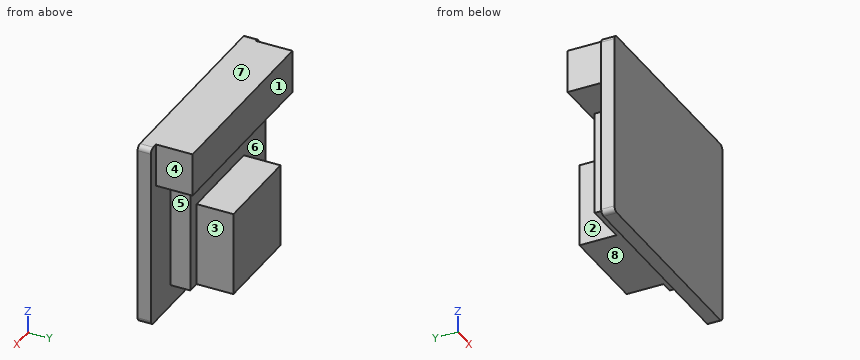
```python
from build123d import *

# Parameters (mm, degrees)
BOSS_EXTRUDE1_DEPTH = 6.5
SKETCH2_W           = 95.29
SKETCH2_H           = 21.2
BOSS_EXTRUDE2_DEPTH = 17.9
SKETCH3_W           = 71.45
SKETCH3_H           = 51
BOSS_EXTRUDE3_DEPTH = 9.77
SKETCH4_W           = 44.95
SKETCH4_H           = 41.1
BOSS_EXTRUDE4_DEPTH = 18


with BuildPart() as part:
    # Sketch1 → Boss-Extrude1 (new body)
    with BuildSketch(Plane(origin=(0, 0, 0), x_dir=(1, 0, 0), z_dir=(0, 1, 0))):
        with BuildLine():
            Line((-51.5, -42.95), (-51.5, 42.95))
            ThreePointArc((-51.5, 42.95), (-50.826345597, 44.576345597), (-49.2, 45.25))
            Line((-49.2, 45.25), (49.2, 45.25))
            ThreePointArc((49.2, 45.25), (50.826345597, 44.576345597), (51.5, 42.95))
            Line((51.5, 42.95), (51.5, -42.95))
            ThreePointArc((51.5, -42.95), (50.826345597, -44.576345597), (49.2, -45.25))
            Line((49.2, -45.25), (-49.2, -45.25))
            ThreePointArc((-49.2, -45.25), (-50.826345597, -44.576345597), (-51.5, -42.95))
        make_face()
    extrude(amount=BOSS_EXTRUDE1_DEPTH)

    # Sketch2 → Boss-Extrude2 (add)
    with BuildSketch(Plane(origin=(0, 6.5, 0), x_dir=(1, 0, 0), z_dir=(0, 1, 0))):
        with Locations((-1.005, -34.65)):
            Rectangle(SKETCH2_W, SKETCH2_H)
    extrude(amount=BOSS_EXTRUDE2_DEPTH)

    # Sketch3 → Boss-Extrude3 (add)
    with BuildSketch(Plane(origin=(0, 6.5, 0), x_dir=(1, 0, 0), z_dir=(0, 1, 0))):
        with Locations((-2.925, 9.25)):
            Rectangle(SKETCH3_W, SKETCH3_H)
    extrude(amount=BOSS_EXTRUDE3_DEPTH)

    # Sketch4 → Boss-Extrude4 (add)
    with BuildSketch(Plane(origin=(0, 16.27, 0), x_dir=(1, 0, 0), z_dir=(0, 1, 0))):
        with Locations((4.425, 14.2)):
            Rectangle(SKETCH4_W, SKETCH4_H)
    extrude(amount=BOSS_EXTRUDE4_DEPTH)


solid = part.part
```
Build history of the part. All positions in model axes, mm. Face numbers are marked on the shaded views. A direction names the side the tool comes from. Coordinates: 2 decimals unless noted, no trailing zeros. Write each loop counter-clockwise with the first axis right and the second up, starting at its lowest first coordinate (ties: lowest second). Pieces come first, ordered by that corner, then holes.
1. Drill centre lines: probe 1 along Z at (x, y) = (-20.5, 15.5); probe 2 along Z at (x, y) = (15.5, 22); probe 3 along Y at (x, z) = (44.5, 38.5). Where is each one in solid material? Low to high.
Answer block:
probe 1: z = -34.75 to 16.25, 24.05 to 45.25
probe 2: z = -34.75 to 6.35, 24.05 to 45.25
probe 3: y = 0 to 24.4
2. Drop flat-ended pins along their axis: pin 1 (5.5 mm diameter, centred on x = -17.5, y = 13, fed in from -Z); pin 2 (6.5 mm diameter, centred on x = 20.5, z = 39.5, fed in from +Y); pin 3 (8 mm diameter, centred on y = 12.5, z = -15, fed in from +X). Give the stop position or say it passes through.
Answer block:
pin 1: stops at z = -34.75
pin 2: stops at y = 24.4
pin 3: stops at x = 32.8
3. Band-saw the part on B-B, the plane z = 12. Give the cut face in (x, y), and give its area (3 significant figures).
Answer block:
outline: (-51.5, 0) - (51.5, 0) - (51.5, 6.5) - (32.8, 6.5) - (32.8, 16.27) - (-38.65, 16.27) - (-38.65, 6.5) - (-51.5, 6.5) - close
area: 1,370 mm2
4. 3-axis set-ups, long thin cutter, end or side, ignore diameter. For the marked faces 1, 2, 3 and 4: which of +Z, -Z, +X, -X, +Y, -Y reach the whole face in a straight line?
Answer block:
face 1: +Z, +X, -X, +Y
face 2: -Z, -X, +Y
face 3: -Z, +X, +Y
face 4: +Z, -Z, +X, +Y
5. Pull direction Z, two halves, no side cores. Call the marked faces 5, 6, 7 and 8: released by +Z, released by -Z, zero draft, split by the parting line, or undercut.
Answer block:
face 5: zero draft
face 6: undercut
face 7: released by +Z
face 8: released by -Z
6. Band-saw the part on A-A, the plane y = 22. Give the cut face in (x, z).
Answer block:
outline: (-48.65, 24.05) - (46.64, 24.05) - (46.64, 45.25) - (-48.65, 45.25) - close; (-18.05, -34.75) - (26.9, -34.75) - (26.9, 6.35) - (-18.05, 6.35) - close
7. Band-saw the part on C-C, the plane x = 38. Give the cut face in (y, z).
Answer block:
outline: (0, -45.25) - (6.5, -45.25) - (6.5, 24.05) - (24.4, 24.05) - (24.4, 45.25) - (0, 45.25) - close
8. Band-saw the part on D-D, the plane y = 11.5. Give the cut face in (x, z), and give its area (3 significant figures).
Answer block:
outline: (-48.65, 24.05) - (46.64, 24.05) - (46.64, 45.25) - (-48.65, 45.25) - close; (-38.65, -34.75) - (32.8, -34.75) - (32.8, 16.25) - (-38.65, 16.25) - close
area: 5,660 mm2
